```python
from build123d import *

# Parameters (mm, degrees)
SKETCH2_R           = 2.625
BOSS_EXTRUDE1_DEPTH = 14
SKETCH3_R           = 9
BOSS_EXTRUDE2_DEPTH = 8
SKETCH4_R           = 2.5
CUT_EXTRUDE1_DEPTH  = 23
CHAMFER1_SIZE       = 2
CUT_EXTRUDE2_DEPTH  = 2.7
CUT_EXTRUDE3_REACH  = 20
SKETCH7_R           = 1.65
CHAMFER2_SIZE       = 0.5
CHAMFER3_SIZE       = 0.5


with BuildPart() as part:
    # Sketch2 → Boss-Extrude1 (new body)
    with BuildSketch(Plane.XY):
        Polygon((4.873707771, 0), (4.832012177, -0.636146486), (4.707640171, -1.261407971), (4.502718925, -1.865087032), (5.52904892, -2.817190886), (5.281517029, -3.257688046), (4.998967171, -3.676585913), (4.683272839, -4.071106911), (3.44623208, -3.44623208), (2.966924906, -3.866571903), (2.436853886, -4.2207551), (1.865087032, -4.502718925), (1.917572975, -5.901682854), (1.431063056, -6.038129807), (0.935064673, -6.134541988), (0.432866603, -6.190280914), (0, -4.873707771), (-0.636146486, -4.832012177), (-1.261407971, -4.707640171), (-1.865087032, -4.502718925), (-2.817190886, -5.52904892), (-3.257688046, -5.281517029), (-3.676585913, -4.998967171), (-4.071106911, -4.683272839), (-3.44623208, -3.44623208), (-3.866571903, -2.966924906), (-4.2207551, -2.436853886), (-4.502718925, -1.865087032), (-5.901682854, -1.917572975), (-6.038129807, -1.431063056), (-6.134541988, -0.935064673), (-6.190280914, -0.432866603), (-4.873707771, 0), (-4.832012177, 0.636146486), (-4.707640171, 1.261407971), (-4.502718925, 1.865087032), (-5.52904892, 2.817190886), (-5.281517029, 3.257688046), (-4.998967171, 3.676585913), (-4.683272839, 4.071106911), (-3.44623208, 3.44623208), (-2.966924906, 3.866571903), (-2.436853886, 4.2207551), (-1.865087032, 4.502718925), (-1.917572975, 5.901682854), (-1.431063056, 6.038129807), (-0.935064673, 6.134541988), (-0.432866603, 6.190280914), (0, 4.873707771), (0.636146486, 4.832012177), (1.261407971, 4.707640171), (1.865087032, 4.502718925), (2.817190886, 5.52904892), (3.257688046, 5.281517029), (3.676585913, 4.998967171), (4.071106911, 4.683272839), (3.44623208, 3.44623208), (3.866571903, 2.966924906), (4.2207551, 2.436853886), (4.502718925, 1.865087032), (5.901682854, 1.917572975), (6.038129807, 1.431063056), (6.134541988, 0.935064673), (6.190280914, 0.432866603), align=None)
        Circle(SKETCH2_R, mode=Mode.SUBTRACT)
    extrude(amount=BOSS_EXTRUDE1_DEPTH)

    # Sketch3 → Boss-Extrude2 (add)
    with BuildSketch(Plane(origin=(0, 0, 0), x_dir=(-1, 0, 0), z_dir=(0, 0, -1))):
        Circle(SKETCH3_R)
    extrude(amount=BOSS_EXTRUDE2_DEPTH)

    # Sketch4 → Cut-Extrude1 (cut, through all)
    with BuildSketch(Plane(origin=(0, 0, -8), x_dir=(-1, 0, 0), z_dir=(0, 0, -1))):
        Circle(SKETCH4_R)
    extrude(amount=-CUT_EXTRUDE1_DEPTH, mode=Mode.SUBTRACT)

    # Sketch5 → Revolve1 (revolve)
    with BuildSketch(Plane(origin=(0, 0, 0), x_dir=(1, 0, 0), z_dir=(0, 1, 0))):
        Polygon((2.5, -14), (7, -14), (7, -13.2), (2.5, -11), align=None)
    revolve(axis=Axis((0, 0, 0), (0, 0, 1)))

    # Chamfer1
    chamfer1_edges = [part.edges().sort_by_distance(p)[0] for p in [
        (9, 0, 0),
    ]]
    chamfer(chamfer1_edges, length=CHAMFER1_SIZE)

    # Sketch6 → Cut-Extrude2 (cut)
    with BuildSketch(Plane(origin=(4, 0, 0), x_dir=(0, 0, -1), z_dir=(1, 0, 0))):
        Polygon((8, 2.9), (8, -2.9), (3.325684219, -2.9), (1.651368439, 0), (3.325684219, 2.9), align=None)
    extrude(amount=CUT_EXTRUDE2_DEPTH, mode=Mode.SUBTRACT)

    # Cut-Extrude3: up to this face of the body
    cut_extrude3_end = part.part.faces().sort_by_distance((2.5, 0, -4))[0]
    # Sketch7 → Cut-Extrude3 (cut, up to the picked face)
    with BuildSketch(Plane(origin=(9, 0, 0), x_dir=(0, 0, -1), z_dir=(1, 0, 0)), mode=Mode.PRIVATE) as cut_extrude3_sk1:
        with Locations((5, 0)):
            Circle(SKETCH7_R)
    cut_extrude3_tool1 = split(extrude(cut_extrude3_sk1.sketch, amount=-CUT_EXTRUDE3_REACH, mode=Mode.PRIVATE), bisect_by=cut_extrude3_end, keep=Keep.BOTH, mode=Mode.PRIVATE)
    add(cut_extrude3_tool1.solids().sort_by_distance((9, 0, -5))[0], mode=Mode.SUBTRACT)

    # Chamfer2
    chamfer2_edges = [part.edges().sort_by_distance(p)[0] for p in [
        (5.35, 2.9, -8),
        (5.35, -2.9, -8),
    ]]
    chamfer(chamfer2_edges, length=CHAMFER2_SIZE)

    # Chamfer3
    chamfer3_edges = [part.edges().sort_by_distance(p)[0] for p in [
        (2.5, 0, -8),
    ]]
    chamfer(chamfer3_edges, length=CHAMFER3_SIZE)


solid = part.part
```
Build history of the part. All positions in model axes, mm. A direction names the side the tool comes from. Give positions to 0.01 mm unless a question says otherwise; leave off trailing zeros. Loops run counter-clockwise (first coordinate to the right, second up) from the corner with the lowest first, then second, coordinate; pieces in that order, holes last. Notation, with made-up numbers: (77.5, 49) -> (117.5, 49) arc R26 cw to (117.5, 72) -> close; hole circle Ø8 at (24.5, -21.5). An arc over 180 degrees is marked (long way). One line per question, with ' | ' between items. Start each with the question number.
1) 3-axis set-ups, long thin cutter, end or side, ignore diameter. For faces 5 (the flat face through (5, 2.9, -5)), 6 (the flat face through (5.19, 1.89, 6.32)), 7 (the flat face through (-1.89, 5.19, 6.32)), 8 (the flat face through (5.54, 0.22, 6.32)): which of +Z, -Z, +X, -X, +Y, -Y reach the whole face in a straight line?
2) Probe L1, parallel to X at y = 0, z = -2.75; L2, parallel to Z at x = 3.5, y = 0; L3, parallel to Z at x = 0.75, y = 5. List the from-to ranges inside material, lowest first.
3) Two-plate mould, pull along X, no slides. Class faces 1 (the conical face through (1.54, -6.96, -0.13)), 2 (the flat face through (-4.07, 3.76, 6.32)), 3 (the flat face through (-3.76, -4.07, 6.32)), 4 (the flat face through (1.89, -5.19, 6.32)): released by +X, released by -X, zero draft, split by the parting line, or undercut.
4) Pin check, flat tips, straight feed: pin 1 (5 mm diameter, centred on y = -5.5, z = -4.5, fed in from +X); pin 2 (1.5 mm diameter, centred on x = -5.5, z = 2, fed in from +Y); pin 3 (2 mm diameter, centred on x = 5, z = -4.5, fed in from -Y). Stop position of each tip, or through.
5) Cut at A-A (z = -5). Give the cut face in (x, y), plus the area to 3 significant figures.
Return value:
1) face 5: -Z | face 6: +Y | face 7: -X | face 8: +X
2) L1: -9 to -2.5, 2.5 to 4, 6.7 to 9 | L2: -8 to -6.65, -3.35 to 14 | L3: -8 to 0, 12.25 to 14
3) face 1: split by the parting line | face 2: undercut | face 3: released by -X | face 4: released by +X
4) pin 1: x = 8.49 | pin 2: y = 3.99 | pin 3: y = -8.06
5) outline: (1.88, -1.65) arc R2.5 cw (long way) to (1.88, 1.65) -> (4, 1.65) -> (4, 2.9) -> (6.7, 2.9) -> (6.7, 1.65) -> (8.85, 1.65) arc R9 ccw (long way) to (8.85, -1.65) -> (6.7, -1.65) -> (6.7, -2.9) -> (4, -2.9) -> (4, -1.65) -> close | area: 206 mm^2
